Input: part model. Units: mm. Frame: model coordinates. A direction names the side the tool comes from. Coordinates: 2 decimals unless noted, no trailing zeros. Loops run counter-clockwise (first coordinate to the right, second up) from the corner with the lowest first, then second, coordinate; pieces in that order, holes last. Notation, with made-up numbers: (-13, -28.75) - (30, -28.75) arc R15 ccw to (30, -4.75) - close; hole circle Ø1 at (9, -20). An arc over 180 degrees is marked (long way). Use a Markdown table: item, result. Add a question column.
1. Contact query for flat-ended pins moving along their axis: P1, Ø3, axis at y = 13, z = -46.5, coming from the -X side; P2, Ø8, axis at x = 24, z = -30, coming from the +Y side; P3, Ø0.6, axis at x = 27, y = 7, coming from the -Z side; P4, Ø5, axis at x = 1, y = 10, coming from the -Z side. Output: stop coordinate, or through.
2. Section query B-B on x = 7. State how many separate pieces and enclosed holes the cut face has, then the cut area to 3 significant figures.
3. Section query A-A on z = -25.5. Return the cut outline in (x, y).
4. Draft query along X for faces 1 (the face through (29, -1, -27)), 2 (the face through (14.297, 31.996, -41.834)), 3 (the face through (4, -2, -21)). Return one class per face: released by +X, released by -X, zero draft, split by the parting line, or undercut.
5. Access query for faces 4 (the face through (16, 10, -41.9)), 5 (the face through (13, 0.5, 2)), 6 (the face through (14, -2, -1)), 7 (the face through (14, 26, -38.9)). Directions: +Z, -Z, +X, -X, +Y, -Y. A direction counts if a zero-diameter tool reaches every point of the face in a straight line with its end or side. Return the directions, or none.
6. Ray query, L1, parallel to Y at x = 1.25, z = -38.52 (3 decimals); L2, parallel to Z at x = 1, y = 17; L3, parallel to Z at x = 13.5, y = 2. Return the intervals inside material, ascending. Write a range as [from, to].
```python
from build123d import *

# Parameters (mm, degrees)
SKETCH1_W            = 41.9
SKETCH1_H            = 21
SKETCH1_R            = 1.125
BOSS_EXTRUDE1_DEPTH  = 3
SKETCH1_3_W          = 47.9
SKETCH1_3_H          = 27
SKETCH1_3_W_2        = 41.9
SKETCH1_3_H_2        = 21
BOSS_EXTRUDE2_DEPTH  = 29
CUT_EXTRUDE1_REACH   = 62.921
SKETCH2_W            = 15
SKETCH2_H            = 20
SKETCH4_W            = 21
SKETCH4_H            = 39.9
CUT_EXTRUDE2_DEPTH   = 35
SKETCH5_R            = 4
BOSS_EXTRUDE3_DEPTH  = 4
SKETCH6_W            = 4
SKETCH6_H            = 27
BOSS_EXTRUDE4_DEPTH  = 6.55
SKETCH7_W            = 4
SKETCH7_H            = 27
BOSS_EXTRUDE5_DEPTH  = 6.55
CUT_EXTRUDE3_REACH   = 67.667
SKETCH10_R           = 2
BOSS_EXTRUDE10_REACH = 65.75
SKETCH11_R           = 1.5
FILLET3_SIZE         = 10
FILLET3_SIZE_2       = 6
CUT_EXTRUDE4_REACH   = 73.257
SKETCH12_R           = 1.5


with BuildPart() as part:
    # Sketch1 → Boss-Extrude1 (new body)
    with BuildSketch(Plane(origin=(0, 0, 0), x_dir=(0, 0, -1), z_dir=(1, 0, 0))):
        with Locations((20.95, 10.5)):
            Rectangle(SKETCH1_W, SKETCH1_H)
        with Locations((38.52, 17.62)):
            Circle(SKETCH1_R, mode=Mode.SUBTRACT)
        with Locations((38.52, 3.38)):
            Circle(SKETCH1_R, mode=Mode.SUBTRACT)
        with Locations((3.38, 17.62)):
            Circle(SKETCH1_R, mode=Mode.SUBTRACT)
        with Locations((3.38, 3.38)):
            Circle(SKETCH1_R, mode=Mode.SUBTRACT)
    extrude(amount=BOSS_EXTRUDE1_DEPTH)

    # Sketch1<3> → Boss-Extrude2 (add)
    with BuildSketch(Plane(origin=(0, 0, 0), x_dir=(0, 0, -1), z_dir=(1, 0, 0))):
        with Locations((20.95, 10.5)):
            Rectangle(SKETCH1_3_W, SKETCH1_3_H)
        with Locations((20.95, 10.5)):
            Rectangle(SKETCH1_3_W_2, SKETCH1_3_H_2, mode=Mode.SUBTRACT)
    extrude(amount=BOSS_EXTRUDE2_DEPTH)

    # Sketch2 → Cut-Extrude1 (cut, up to next)
    with BuildSketch(Plane.XY.offset(3), mode=Mode.PRIVATE) as cut_extrude1_sk1:
        with Locations((13.3, 10.5)):
            Rectangle(SKETCH2_W, SKETCH2_H)
    cut_extrude1_tool1 = extrude(cut_extrude1_sk1.sketch, amount=-CUT_EXTRUDE1_REACH, mode=Mode.PRIVATE) & part.part
    add(cut_extrude1_tool1.solids().sort_by_distance((13.3, 10.5, 3))[0], mode=Mode.SUBTRACT)

    # Sketch4 → Cut-Extrude2 (cut)
    with BuildSketch(Plane.XZ.offset(3)):
        with Locations((14.5, -20.95)):
            Rectangle(SKETCH4_W, SKETCH4_H)
    extrude(amount=-CUT_EXTRUDE2_DEPTH, mode=Mode.SUBTRACT)

    # Sketch5 → Boss-Extrude3 (add)
    with BuildSketch(Plane.ZY):
        with Locations(Location((-10.5, 10.5, 0), (0, 0, 180))):
            Circle(SKETCH5_R)
    extrude(amount=BOSS_EXTRUDE3_DEPTH)

    # Sketch6 → Boss-Extrude4 (add)
    with BuildSketch(Plane(origin=(0, 0, -44.9), x_dir=(-1, 0, 0), z_dir=(0, 0, -1))):
        with Locations((-27, 10.5)):
            Rectangle(SKETCH6_W, SKETCH6_H)
    extrude(amount=BOSS_EXTRUDE4_DEPTH)

    # Sketch7 → Boss-Extrude5 (add)
    with BuildSketch(Plane.XY.offset(3)):
        with Locations((27, 10.5)):
            Rectangle(SKETCH7_W, SKETCH7_H)
    extrude(amount=BOSS_EXTRUDE5_DEPTH)

    # Sketch10 → Cut-Extrude3 (cut, up to next)
    with BuildSketch(Plane(origin=(29, 0, 0), x_dir=(0, 0, -1), z_dir=(1, 0, 0)), mode=Mode.PRIVATE) as cut_extrude3_sk1:
        with Locations((-3.35, 15.5)):
            Circle(SKETCH10_R)
    cut_extrude3_tool1 = extrude(cut_extrude3_sk1.sketch, amount=-CUT_EXTRUDE3_REACH, mode=Mode.PRIVATE) & part.part
    # Sketch10 → Cut-Extrude3 (cut, up to next)
    with BuildSketch(Plane(origin=(29, 0, 0), x_dir=(0, 0, -1), z_dir=(1, 0, 0)), mode=Mode.PRIVATE) as cut_extrude3_sk2:
        with Locations((-3.35, 5.5)):
            Circle(SKETCH10_R)
    cut_extrude3_tool2 = extrude(cut_extrude3_sk2.sketch, amount=-CUT_EXTRUDE3_REACH, mode=Mode.PRIVATE) & part.part
    # Sketch10 → Cut-Extrude3 (cut, up to next)
    with BuildSketch(Plane(origin=(29, 0, 0), x_dir=(0, 0, -1), z_dir=(1, 0, 0)), mode=Mode.PRIVATE) as cut_extrude3_sk3:
        with Locations((45.25, 5.5)):
            Circle(SKETCH10_R)
    cut_extrude3_tool3 = extrude(cut_extrude3_sk3.sketch, amount=-CUT_EXTRUDE3_REACH, mode=Mode.PRIVATE) & part.part
    # Sketch10 → Cut-Extrude3 (cut, up to next)
    with BuildSketch(Plane(origin=(29, 0, 0), x_dir=(0, 0, -1), z_dir=(1, 0, 0)), mode=Mode.PRIVATE) as cut_extrude3_sk4:
        with Locations((45.25, 15.5)):
            Circle(SKETCH10_R)
    cut_extrude3_tool4 = extrude(cut_extrude3_sk4.sketch, amount=-CUT_EXTRUDE3_REACH, mode=Mode.PRIVATE) & part.part
    add(cut_extrude3_tool1.solids().sort_by_distance((29, 15.5, 3.35))[0], mode=Mode.SUBTRACT)
    add(cut_extrude3_tool2.solids().sort_by_distance((29, 5.5, 3.35))[0], mode=Mode.SUBTRACT)
    add(cut_extrude3_tool3.solids().sort_by_distance((29, 5.5, -45.25))[0], mode=Mode.SUBTRACT)
    add(cut_extrude3_tool4.solids().sort_by_distance((29, 15.5, -45.25))[0], mode=Mode.SUBTRACT)

    # Boss-Extrude10: up to this face of the body (flat: up to its plane)
    boss_extrude10_end = Plane(part.part.faces().sort_by_distance((29, 10.5, -50.782916797))[0])
    # Sketch11 → Boss-Extrude10 (add, up to the picked face)
    with BuildSketch(Plane.ZY, mode=Mode.PRIVATE) as boss_extrude10_sk1:
        with BuildLine():
            Line((-44.9, 29), (-44.9, 24))
            Line((-44.9, 24), (-38.9, 24))
            Line((-38.9, 24), (-38.9, 29))
            Line((-38.9, 29), (-38.903642649, 29))
            ThreePointArc((-38.903642649, 29), (-41.9, 31.996357351), (-44.896357351, 29))
            Line((-44.896357351, 29), (-44.9, 29))
        make_face()
        with Locations((-41.9, 29)):
            Circle(SKETCH11_R, mode=Mode.SUBTRACT)
    boss_extrude10_tool1 = split(extrude(boss_extrude10_sk1.sketch, amount=-BOSS_EXTRUDE10_REACH, mode=Mode.PRIVATE), bisect_by=boss_extrude10_end, keep=Keep.BOTH, mode=Mode.PRIVATE)
    # Sketch11 → Boss-Extrude10 (add, up to the picked face)
    with BuildSketch(Plane.ZY, mode=Mode.PRIVATE) as boss_extrude10_sk2:
        with BuildLine():
            Line((-44.9, 7.530863133), (-44.9, 13.530863133))
            Line((-44.9, 13.530863133), (-51.45, 13.530863133))
            ThreePointArc((-51.45, 13.530863133), (-54.45, 10.530863133), (-51.45, 7.530863133))
            Line((-51.45, 7.530863133), (-44.9, 7.530863133))
        make_face()
        with Locations((-51.45, 10.530863133)):
            Circle(SKETCH11_R, mode=Mode.SUBTRACT)
    boss_extrude10_tool2 = split(extrude(boss_extrude10_sk2.sketch, amount=-BOSS_EXTRUDE10_REACH, mode=Mode.PRIVATE), bisect_by=boss_extrude10_end, keep=Keep.BOTH, mode=Mode.PRIVATE)
    # Sketch11 → Boss-Extrude10 (add, up to the picked face)
    with BuildSketch(Plane.ZY, mode=Mode.PRIVATE) as boss_extrude10_sk3:
        with BuildLine():
            Line((-38.9, -3), (-44.9, -3))
            Line((-44.9, -3), (-44.9, -7.358406619))
            ThreePointArc((-44.9, -7.358406619), (-41.9, -11.067839968), (-38.9, -7.358406619))
            Line((-38.9, -7.358406619), (-38.9, -3))
        make_face()
        with Locations((-41.9, -8)):
            Circle(SKETCH11_R, mode=Mode.SUBTRACT)
    boss_extrude10_tool3 = split(extrude(boss_extrude10_sk3.sketch, amount=-BOSS_EXTRUDE10_REACH, mode=Mode.PRIVATE), bisect_by=boss_extrude10_end, keep=Keep.BOTH, mode=Mode.PRIVATE)
    add(boss_extrude10_tool1.solids().sort_by(Axis((0, 27.459117, -41.9), (1, 0, 0)))[0])
    add(boss_extrude10_tool2.solids().sort_by(Axis((0, 10.530863, -49.062446), (1, 0, 0)))[0])
    add(boss_extrude10_tool3.solids().sort_by(Axis((0, -5.179203, -39.001359), (1, 0, 0)))[0])

    # Fillet3
    # an asymmetric fillet: 10, 6 mm, written as the material it takes off along each edge
    with BuildSketch(Plane(origin=(54, 24, 9.55), x_dir=(0, -1, 0), z_dir=(-1, 0, 0)), Plane(origin=(0, 24, -51.45), x_dir=(0, -1, 0), z_dir=(1, 0, 0))) as fillet3_piece_1:
        with BuildLine():
            Bezier((FILLET3_SIZE, 0), (0, 0), (0, -FILLET3_SIZE_2), weights=[1, 0.707106781, 1])
            Line((0, -FILLET3_SIZE_2), (0, 0))
            Line((0, 0), (FILLET3_SIZE, 0))
        make_face()
    extrude(amount=54, mode=Mode.SUBTRACT)
    with BuildSketch(Plane(origin=(0, -3, 9.55), x_dir=(0, 0, -1), z_dir=(1, 0, 0)), Plane(origin=(54, -3, -51.45), x_dir=(0, 0, 1), z_dir=(-1, 0, 0))) as fillet3_piece_2:
        with BuildLine():
            Bezier((FILLET3_SIZE_2, 0), (0, 0), (0, FILLET3_SIZE), weights=[1, 0.707106781, 1])
            Line((0, FILLET3_SIZE), (0, 0))
            Line((0, 0), (FILLET3_SIZE_2, 0))
        make_face()
    extrude(amount=54, mode=Mode.SUBTRACT)

    # Sketch12 → Cut-Extrude4 (cut, up to next)
    with BuildSketch(Plane(origin=(29, 0, 0), x_dir=(0, 0, -1), z_dir=(1, 0, 0)), mode=Mode.PRIVATE) as cut_extrude4_sk1:
        with Locations(Location((51.45, 10.530863133, 0), (0, 0, 180))):
            Circle(SKETCH12_R)
    cut_extrude4_tool1 = extrude(cut_extrude4_sk1.sketch, amount=-CUT_EXTRUDE4_REACH, mode=Mode.PRIVATE) & part.part
    add(cut_extrude4_tool1.solids().sort_by_distance((29, 10.530863, -51.45))[0], mode=Mode.SUBTRACT)


solid = part.part
```
Resolved:
| question | item | result |
|---|---|---|
| 1 | P1 | x = 0 |
| 1 | P2 | y = 24 |
| 1 | P3 | z = -51.45 |
| 1 | P4 | z = -54.45 |
| 2 | separate pieces | 3 |
| 2 | enclosed holes | 3 |
| 2 | area | 225 mm² |
| 3 | outline | (0, -3) - (4, -3) - (4, 0) - (3, 0) - (3, 21) - (4, 21) - (4, 24) - (0, 24) - close; (25, -3) - (29, -3) - (29, 0) - (25, 0) - close; (25, 21) - (29, 21) - (29, 24) - (25, 24) - close |
| 4 | face 1 | released by +X |
| 4 | face 2 | zero draft |
| 4 | face 3 | undercut |
| 5 | face 4 | +X |
| 5 | face 5 | +Z |
| 5 | face 6 | +Y, -Y |
| 5 | face 7 | +Z, +X, -X, +Y |
| 6 | L1 | [-3, 2.255], [4.505, 16.495], [18.745, 24] |
| 6 | L2 | [-43.93, -39.46], [-37.58, -4.32], [-2.44, 3] |
| 6 | L3 | [-44.9, -41.9] |
